Geometry: final body of the model. Coordinates: model frame, mm. Face numbers are marked on the shaded views. Coordinates: 2 decimals unless noted, no trailing zeros. Write each loop counter-clockwise with the first axis right and the second up, starting at its lowest first coordinate (ties: lowest second). Pieces come first, ordered by that corner, then holes.
from build123d import *

# Parameters (mm, degrees)
FILLET1_R = 1


with BuildPart() as part:
    # Sketch1 → Revolve1 (revolve)
    with BuildSketch(Plane.XY):
        with BuildLine():
            Line((0, 11.5), (0, 15.25))
            Line((0, 15.25), (2, 15.25))
            Line((2, 15.25), (5, 13.517949192))
            Line((5, 13.517949192), (5, 11.5))
            Line((5, 11.5), (2.65, 11.5))
            ThreePointArc((2.65, 11.5), (1.75, 11.2), (0.85, 11.5))
            Line((0.85, 11.5), (0, 11.5))
        make_face()
    revolve(axis=Axis((0, 0, 0), (1, 0, 0)))

    # Fillet1
    fillet1_edges = [part.edges().sort_by_distance(p)[0] for p in [
        (0, -15.25, 0),
    ]]
    fillet(fillet1_edges, radius=FILLET1_R)


solid = part.part
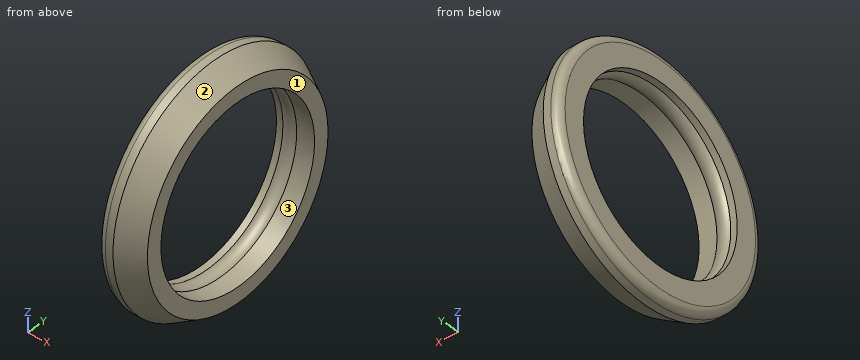
Item 1: Material intervals for probe 1 along Z at (x, y) = (1.1, -10); probe 2 along Z at (x, y) = (0.65, 0); probe 3 along Y at (x, z) = (3.2, 2), sorted ascending.
Derived:
probe 1: z = -11.51 to -5.36, 5.36 to 11.51
probe 2: z = -15.19 to -11.5, 11.5 to 15.19
probe 3: y = -14.42 to -11.32, 11.32 to 14.42
Item 2: Section A-A, the plane z = 0. Output: boundary loops of the cut face in (x, y), plus the area to 3 significant figures.
Derived:
outline: (0, -14.25) arc R1 ccw to (1, -15.25) - (2, -15.25) - (5, -13.52) - (5, -11.5) - (2.65, -11.5) arc R1.5 ccw to (0.85, -11.5) - (0, -11.5) - close; (0, 11.5) - (0.85, 11.5) arc R1.5 ccw to (2.65, 11.5) - (5, 11.5) - (5, 13.52) - (2, 15.25) - (1, 15.25) arc R1 ccw to (0, 14.25) - close
area: 32.6 mm2
Item 3: Section C-C, the plane x = 3.9. Output: boundary loops of the cut face in (y, z).
Derived:
outline: circle Ø28.31 at (0, 0); hole circle Ø23 at (0, 0)
Item 4: Pull-direction query (Z, two-part tool) for the marked faces 1, 2 and 3; classes: released by +Z, released by -Z, zero draft, split by the parting line, or undercut.
Derived:
face 1: zero draft
face 2: split by the parting line
face 3: undercut
Item 5: Pin query (flat end, axial travel): pin 1 (3 mm diameter, centred on y = -12, z = -11.5, fed in from +X); pin 2 (1 mm diameter, centred on x = 1, z = 6, fed in from -Y); pin 3 (1.5 mm diameter, centred on x = 1.5, z = -4.5, fed in from -Y). Return the tip coordinate at first contact, or that it passes through.
Derived:
pin 1: stops at x = 2.22
pin 2: stops at y = -14.22
pin 3: stops at y = -14.78
